```python
from build123d import *

# Parameters (mm, degrees)
SKETCH1_R               = 97.28
SKETCH1_R_2             = 2.8067
SKETCH1_R_3             = 8
BOSS_EXTRUDE1_DEPTH     = 3
F_1_4_CLEARANCE_HOLE1_D = 6.7564


with BuildPart() as part:
    # Sketch1 → Boss-Extrude1 (new body)
    with BuildSketch(Plane.XY):
        with Locations((36.235962131, -23.183312097)):
            Circle(SKETCH1_R)
        with Locations((61.635962131, -7.308312097)):
            Circle(SKETCH1_R_2, mode=Mode.SUBTRACT)
        with Locations((61.635962131, -39.058312097)):
            Circle(SKETCH1_R_2, mode=Mode.SUBTRACT)
        with Locations((10.835962131, -39.058312097)):
            Circle(SKETCH1_R_2, mode=Mode.SUBTRACT)
        with Locations((10.835962131, -7.308312097)):
            Circle(SKETCH1_R_2, mode=Mode.SUBTRACT)
        with Locations((-5.014037869, -64.433312097)):
            Circle(SKETCH1_R_3, mode=Mode.SUBTRACT)
        with Locations((77.485962131, -64.433312097)):
            Circle(SKETCH1_R_3, mode=Mode.SUBTRACT)
        with Locations((77.485962131, 18.066687903)):
            Circle(SKETCH1_R_3, mode=Mode.SUBTRACT)
        with Locations((-5.014037869, 18.066687903)):
            Circle(SKETCH1_R_3, mode=Mode.SUBTRACT)
        Polygon((15.735962131, -35.032829738), (36.247945431, -46.861591696), (56.747945431, -35.012074055), (56.735962131, -11.333794456), (36.223978831, 0.494967501), (15.723978831, -11.35455014), align=None, mode=Mode.SUBTRACT)
    extrude(amount=BOSS_EXTRUDE1_DEPTH)

    # 1/4 Clearance Hole1 (through all)
    with Locations(Plane(origin=(0, 0, 0), x_dir=(-1, 0, 0), z_dir=(0, 0, -1))):
        with Locations((-118.735962131, -23.183312097), (-107.683057943, -64.433312097), (46.264037869, -23.183312097), (35.211133681, -64.433312097), (-77.485962131, -94.63040791), (-36.235962131, -105.683312097), (5.014037869, -94.63040791), (35.211133681, 18.066687903), (5.014037869, 48.263783715), (-36.235962131, 59.316687903), (-77.485962131, 48.263783715), (-107.683057943, 18.066687903)):
            Hole(F_1_4_CLEARANCE_HOLE1_D / 2)


solid = part.part
```
CAD build for the part. Positions are in the model's coordinates, mm. A direction names the side the tool comes from. Round coordinates to 2 decimals unless told otherwise and drop trailing zeros. Write each loop counter-clockwise with the first axis right and the second up, starting at its lowest first coordinate (ties: lowest second). Pieces come first, ordered by that corner, then holes. Notation, with made-up numbers: (65, 4) - (90, 4) arc R13 ccw to (90, 26) - close; hole circle Ø7 at (52.5, 42.5). An arc over 180 degrees is marked (long way). Return JSON: item names as keys, results as strings. Group by question number.
Item 1: Mould opens along X. For faces 1 (the face through (-3.46, -97.63, 1.52)), 2 (the face through (35, 0, 0)), 3 (the face through (129.024, 6.037, 1.479)), 4 (the face through (69.494, 18.418, 1.479)) say: +X half, -X half, draft (parallel to the pull), parting line (faces both ways), or undercut.
Item 2: Flat gauge pins, fed straight in: pin 1 Ø1.5 at (x, z) = (17, 2) entering from -Y; pin 2 Ø1.5 at (x, z) = (14.5, 2.5) entering from -Y. Where does each tip first touch, or does it go through?
Item 3: Band-saw the part on C-C on y = -54. List the corners of the cut face in (x, z).
Item 4: 3-axis set-ups, long thin cutter, end or side, ignore diameter. For faces 5 (the face through (25.848, -40.864, 1.479)), 6 (the face through (35, 0, 3)): which of +Z, -Z, +X, -X, +Y, -Y reach the whole face in a straight line?
Item 5: Probe probe 1 along X at (y, z) = (-70, 2.25); probe 2 along Y at (x, z) = (83, 0.6); probe 3 along X at (y, z) = (23.5, 2.55). List the from-to ranges inside material, lowest first.
Item 6: Band-saw the part on A-A on z = 1.1. State how many separate pieces and enclosed holes the cut face has, plus the area to 3 significant figures.
Item 7: Band-saw the part on B-B on x = -19.5. List the corners of the cut face in (y, z), plus the area to 3 significant figures.
Resolved:
{
 "1": {"face 1": "undercut", "face 2": "draft", "face 3": "parting line", "face 4": "undercut"},
 "2": {"pin 1": "stops at y = -118.69", "pin 2": "stops at y = -118.17"},
 "3": {"outline": "(-56.03, 0) - (128.51, 0) - (128.51, 3) - (-56.03, 3) - close"},
 "4": {"face 5": "+Z, -Z", "face 6": "+Z, +X, -X, +Y, -Y"},
 "5": {"probe 1": "x = -49.04 to -10.76, 0.73 to 71.74, 83.23 to 121.51", "probe 2": "y = -108.49 to -70.23, -58.64 to 12.27, 23.86 to 62.12", "probe 3": "x = -49.11 to -10.89, 0.86 to 71.61, 83.36 to 121.58"},
 "6": {"separate pieces": "1", "enclosed holes": "21", "area": "26,900 mm²"},
 "7": {"outline": "(-102.91, 0) - (56.55, 0) - (56.55, 3) - (-102.91, 3) - close", "area": "478 mm²"}
}
